```python
from build123d import *

# Parameters (mm, degrees)
F0_W      = 31.75
F0_H      = 31.75
F1_DEPTH  = 12.7
F3_D      = 19.05
F4_R      = 14.478
F4_R_2    = 12.7
F5_DEPTH  = 0.889
F6_R      = 14.478
F6_R_2    = 12.7
F7_DEPTH  = 0.889
F9_D      = 1.5875
F9_DEPTH  = 7.62
F9_TIP    = 0.4769331164
F11_D     = 1.5875
F11_DEPTH = 7.62
F11_TIP   = 0.4769331164


with BuildPart() as f1:
    # F0 (on Front) → F1 (new body, symmetric)
    with BuildSketch(Plane.XZ):
        Rectangle(F0_W, F0_H)
    extrude(amount=F1_DEPTH, both=True)

    # F3 (through all)
    with Locations(Plane.XZ.offset(12.7)):
        with Locations((0, 0)):
            Hole(F3_D / 2)

    # F4 (on face) → F5 (cut)
    with BuildSketch(Plane.XZ.offset(12.7)):
        Circle(F4_R)
        Circle(F4_R_2, mode=Mode.SUBTRACT)
    extrude(amount=-F5_DEPTH, mode=Mode.SUBTRACT)

    # F6 (on face) → F7 (cut)
    with BuildSketch(Plane(origin=(0, 12.7, 0), x_dir=(-1, 0, 0), z_dir=(0, 1, 0))):
        Circle(F6_R)
        Circle(F6_R_2, mode=Mode.SUBTRACT)
    extrude(amount=-F7_DEPTH, mode=Mode.SUBTRACT)

    # F9
    with Locations(Plane(origin=(0, 12.7, 0), x_dir=(-1, 0, 0), z_dir=(0, 1, 0))):
        with Locations((-13.335, 13.335), (13.335, 13.335), (13.335, -13.335), (-13.335, -13.335)):
            Hole(F9_D / 2, depth=F9_DEPTH)
            with Locations((0, 0, -(F9_DEPTH + F9_TIP / 2))):  # 118° drill point
                Cone(0, F9_D / 2, F9_TIP, mode=Mode.SUBTRACT)

    # F11
    with Locations(Plane.XZ.offset(12.7)):
        with Locations((-13.335, 13.335), (13.335, 13.335), (13.335, -13.335), (-13.335, -13.335)):
            Hole(F11_D / 2, depth=F11_DEPTH)
            with Locations((0, 0, -(F11_DEPTH + F11_TIP / 2))):  # 118° drill point
                Cone(0, F11_D / 2, F11_TIP, mode=Mode.SUBTRACT)


solid = f1.part
```
Model file for the job. Use its own axes, mm. A direction names the side the tool comes from. Coordinates: 2 decimals unless noted, no trailing zeros. Loops run counter-clockwise (first coordinate to the right, second up) from the corner with the lowest first, then second, coordinate; pieces in that order, holes last. Notation, with made-up numbers: M 38.5,58.25 L 97.5,58.25 A17 cw 97.5,83.25 Z; hole C -0.75,24 d2. An arc over 180 degrees is marked long. Use CSV: the item, a comma, the result in double quotes. Start each with the question number.
1. Band-saw the part on C-C, the plane x = -6. List the corners of the cut face in (y, z) (3 decimals).
2. Band-saw the part on D-D, the plane y = -7.25. Give the number of separate pieces and of enclosed holes in the cut face, then the cut area to 3 significant figures.
3. Band-saw the part on B-B, the plane y = 1.75. List the corners of the cut face in (x, z) (3 decimals).
4. Probe probe 1 along Z at (x, y) = (0, 12.25) (3 decimals); probe 2 along Z at (x, y) = (14, -9.5) (3 decimals); probe 3 along Z at (x, y) = (4, -10.75) (3 decimals). List the from-to ranges inside material, lowest first. Write a range as [from, to].
5. Tool access for faces 1 (the flat face through (0, 0, -15.875)), 2 (the cylindrical face through (-13.762, -8.837, 14.004)), 3 (the cylindrical face through (-13.92, 8.84, 13.87)): list every direction of +Z, -Z, +X, -X, +Y, -Y with a clear straight run to the whole face (end or side of a thin tool).
6. Flat gauge pins, fed straight in: pin 1 (2.5 mm diameter, centred on x = -13.335, z = 13.335, fed in from -Y); pin 2 (1.3 mm diameter, centred on x = -13.335, z = 13.335, fed in from +Y). Where does each tip first touch, or does it go through?
7. Band-saw the part on A-A, the plane z = 0. List the corners of the cut face in (x, y) (3 decimals), then the cut area to 3 significant figures.
8. Two-plate mould, pull along X, no slides. Class faces 4 (the flat face through (-5, 12.7, 14)), 5 (the conical face through (13.462, -4.686, 13.282)), 6 (the flat face through (15.875, 0, 0)): pulls with the +X half, pulls with the -X half, needs draft (parallel to the pull), parting line crosses it, or undercut.
Entries:
1,outline,"M -12.7,-15.875 L 12.7,-15.875 L 12.7,-13.176 L 11.811,-13.176 L 11.811,-11.193 L 12.7,-11.193 L 12.7,-7.398 L -12.7,-7.398 L -12.7,-11.193 L -11.811,-11.193 L -11.811,-13.176 L -12.7,-13.176 Z; M -12.7,7.398 L 12.7,7.398 L 12.7,11.193 L 11.811,11.193 L 11.811,13.176 L 12.7,13.176 L 12.7,15.875 L -12.7,15.875 L -12.7,13.176 L -11.811,13.176 L -11.811,11.193 L -12.7,11.193 Z"
2,separate pieces,"1"
2,enclosed holes,"5"
2,area,"715 mm2"
3,outline,"M -15.875,-15.875 L 15.875,-15.875 L 15.875,15.875 L -15.875,15.875 Z; hole C 0,0 d19.05"
4,probe 1,"z = [-15.875, -14.478], [-12.7, -9.525], [9.525, 12.7], [14.478, 15.875]"
4,probe 2,"z = [-15.875, -13.768], [-12.902, 12.902], [13.768, 15.875]"
4,probe 3,"z = [-15.875, -8.644], [8.644, 15.875]"
5,face 1,"-Z, +X, -X, +Y, -Y"
5,face 2,"-Y"
5,face 3,"+Y"
6,pin 1,"stops at y = -12.7"
6,pin 2,"stops at y = 4.99"
7,outline,"M -15.875,-12.7 L -14.478,-12.7 L -14.478,-11.811 L -12.7,-11.811 L -12.7,-12.7 L -9.525,-12.7 L -9.525,12.7 L -12.7,12.7 L -12.7,11.811 L -14.478,11.811 L -14.478,12.7 L -15.875,12.7 Z; M 9.525,-12.7 L 12.7,-12.7 L 12.7,-11.811 L 14.478,-11.811 L 14.478,-12.7 L 15.875,-12.7 L 15.875,12.7 L 14.478,12.7 L 14.478,11.811 L 12.7,11.811 L 12.7,12.7 L 9.525,12.7 Z"
7,area,"316 mm2"
8,face 4,"needs draft"
8,face 5,"undercut"
8,face 6,"pulls with the +X half"
